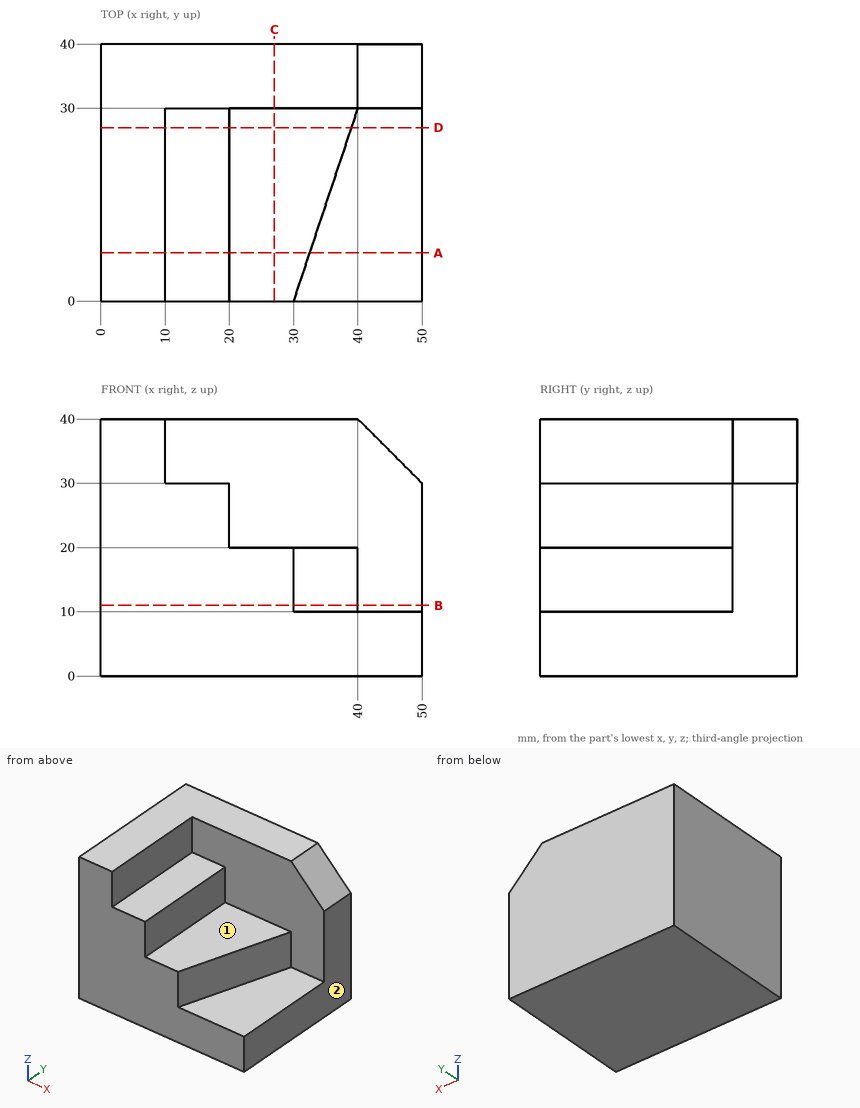
Geometry: see drawing. Coordinates: mm, zero at the bounding-box minimum. A direction names the side the tool comes from. Coordinates: 2 decimals unless noted, no trailing zeros. Loops run counter-clockwise (first coordinate to the right, second up) from the corner with the lowest first, then second, coordinate; pieces in that order, holes last. Notation, with made-up numbers: (-37.75, 44.5) - (10.25, 44.5) arc R10 cw to (10.25, 58.5) - close; hole circle Ø10 at (1, 77.25). An arc over 180 degrees is marked (long way). Put each result on its own line as item: value. Start each with the question number.
Q1. Cut plane B-B, the plane z = 11. Return loops of the section in (x, y), and give its area (3 significant figures).
Q2. Set-up query: the marked faces 1 and 2. Return all of +Z, -Z, +X, -X, +Y, -Y with unobstructed straight access to the full face (end or side cutting, diameter ignored); none if empty.
Q3. Line query: line 1 (X direction, y = 7, z = 29.5); line 2 (Y direction, x = 27.5, z = 26); line 3 (Z direction, x = 41.5, y = 18). Output: solid intervals per line, ascending.
Q4. Cut plane C-C, the plane x = 27. Return loops of the section in (y, z).
Q5. Cut plane A-A, the plane y = 7.5. Return loops of the section in (x, z), and give its area (4 significant figures).
Q6. Pin query (flat end, axial travel): pin 1 Ø11 at (y, z) = (17.5, 22.5) entering from +X; pin 2 Ø3 at (x, y) = (16.5, 21.5) entering from +Z; pin 3 Ø6 at (x, y) = (43, 13.5) entering from -Z; pin 4 Ø12 at (y, z) = (6, 29.5) entering from +X. Return the tip coordinate at first contact, or that it passes through.
Q7. Cut plane D-D, the plane y = 27. Return loops of the section in (x, z).
Filled sheet:
1. outline: (0, 0) - (30, 0) - (40, 30) - (50, 30) - (50, 40) - (0, 40) - close
1. area: 1,550 mm²
2. face 1: +Z, +X, -Y
2. face 2: +Z, -Z, +X, +Y, -Y
3. line 1: 0 to 20
3. line 2: 30 to 40
3. line 3: 0 to 10
4. outline: (0, 0) - (40, 0) - (40, 40) - (30, 40) - (30, 20) - (0, 20) - close
5. outline: (0, 0) - (50, 0) - (50, 10) - (32.5, 10) - (32.5, 20) - (20, 20) - (20, 30) - (10, 30) - (10, 40) - (0, 40) - close
5. area: 1,125 mm²
6. pin 1: x = 37.47
6. pin 2: z = 30
6. pin 3: z = 0
6. pin 4: x = 20
7. outline: (0, 0) - (50, 0) - (50, 10) - (39, 10) - (39, 20) - (20, 20) - (20, 30) - (10, 30) - (10, 40) - (0, 40) - close
